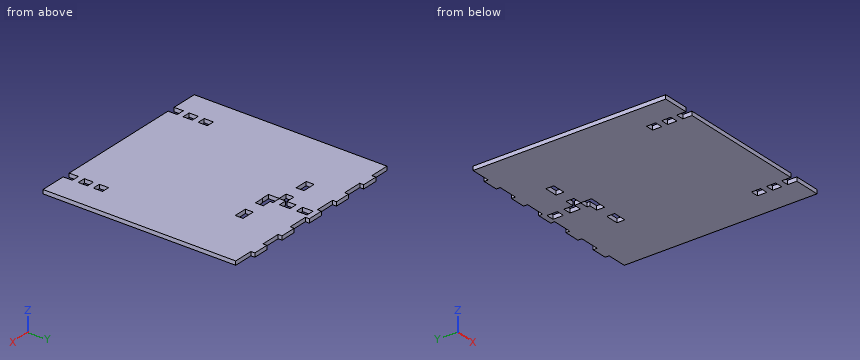
from build123d import *

# Parameters (mm, degrees)
ESQUISSE1_W              = 150
ESQUISSE1_H              = 150
BOSS_EXTRU_1_DEPTH       = 3
ESQUISSE12_W             = 6
ESQUISSE12_H             = 7
ENL_V_MAT_EXTRU_3_DEPTH  = 3
ESQUISSE14_W             = 15
ESQUISSE14_H             = 3
ENL_V_MAT_EXTRU_4_DEPTH  = 3
ESQUISSE15_W             = 10
ESQUISSE15_H             = 6
ESQUISSE15_W_2           = 6
ESQUISSE15_H_2           = 8
ESQUISSE15_W_3           = 7
ENL_V_MAT_EXTRU_9_DEPTH  = 10
ESQUISSE17_W             = 6.4
ESQUISSE17_H             = 8.4
ENL_V_MAT_EXTRU_12_DEPTH = 10


with BuildPart() as part:
    # Esquisse1 → Boss.-Extru.1 (new body)
    with BuildSketch(Plane.XY):
        with Locations((75, -75)):
            Rectangle(ESQUISSE1_W, ESQUISSE1_H)
    extrude(amount=BOSS_EXTRU_1_DEPTH)

    # Esquisse12 → Enlèv. mat.-Extru.3 (cut)
    with BuildSketch(Plane(origin=(0, 0, 0), x_dir=(-1, 0, 0), z_dir=(0, 0, -1))):
        with Locations((-127, -123.5)):
            Rectangle(ESQUISSE12_W, ESQUISSE12_H)
        with Locations((-127, -135)):
            Rectangle(ESQUISSE12_W, ESQUISSE12_H)
        with Locations((-127, -146.5)):
            Rectangle(ESQUISSE12_W, ESQUISSE12_H)
        with Locations((-23, -123.5)):
            Rectangle(ESQUISSE12_W, ESQUISSE12_H)
        with Locations((-23, -135)):
            Rectangle(ESQUISSE12_W, ESQUISSE12_H)
        with Locations((-23, -146.5)):
            Rectangle(ESQUISSE12_W, ESQUISSE12_H)
    extrude(amount=-ENL_V_MAT_EXTRU_3_DEPTH, mode=Mode.SUBTRACT)

    # Esquisse14 → Enlèv. mat.-Extru.4 (cut)
    with BuildSketch(Plane(origin=(0, 0, 0), x_dir=(-1, 0, 0), z_dir=(0, 0, -1))):
        with Locations((-142.5, -1.5)):
            Rectangle(ESQUISSE14_W, ESQUISSE14_H)
        with Locations((-115.5, -1.5)):
            Rectangle(ESQUISSE14_W, ESQUISSE14_H)
        with Locations((-88.5, -1.5)):
            Rectangle(ESQUISSE14_W, ESQUISSE14_H)
        with Locations((-61.5, -1.5)):
            Rectangle(ESQUISSE14_W, ESQUISSE14_H)
        with Locations((-34.5, -1.5)):
            Rectangle(ESQUISSE14_W, ESQUISSE14_H)
        with Locations((-7.5, -1.5)):
            Rectangle(ESQUISSE14_W, ESQUISSE14_H)
    extrude(amount=-ENL_V_MAT_EXTRU_4_DEPTH, mode=Mode.SUBTRACT)

    # Esquisse15 → Enlèv. mat.-Extru.9 (cut)
    with BuildSketch(Plane(origin=(0, 0, 0), x_dir=(-1, 0, 0), z_dir=(0, 0, -1))):
        with Locations((-50, -27)):
            Rectangle(ESQUISSE15_W, ESQUISSE15_H)
        Polygon((-78, -17), (-78, -25), (-72, -25), (-72, -30), (-65, -30), (-65, -24), (-72, -24), (-72, -17), align=None)
        with Locations((-75, -8)):
            Rectangle(ESQUISSE15_W_2, ESQUISSE15_H_2)
        with Locations((-81.5, -35)):
            Rectangle(ESQUISSE15_W_3, ESQUISSE15_H)
        with Locations((-100, -35)):
            Rectangle(ESQUISSE15_W, ESQUISSE15_H)
    extrude(amount=-ENL_V_MAT_EXTRU_9_DEPTH, mode=Mode.SUBTRACT)

    # Esquisse17 → Enlèv. mat.-Extru.12 (cut)
    with BuildSketch(Plane(origin=(0, 0, 0), x_dir=(-1, 0, 0), z_dir=(0, 0, -1))):
        with Locations((-75, -34)):
            Rectangle(ESQUISSE17_W, ESQUISSE17_H)
    extrude(amount=-ENL_V_MAT_EXTRU_12_DEPTH, mode=Mode.SUBTRACT)


solid = part.part
Read the model definition and answer for the solid it produces. Units are mm, in the model's axes. Round coordinates to 2 decimals unless told otherwise and drop trailing zeros. Write each loop counter-clockwise with the first axis right and the second up, starting at its lowest first coordinate (ties: lowest second). Pieces come first, ordered by that corner, then holes.
1. The part is cut by section C-C, the plane x = 138. Determine the outline of the cut face in (y, z).
2. Straight lines are drawn through the part: L1, parallel to X at y = -37, z = 1.2; L2, parallel to X at y = -9.5, z = 2.75; L3, parallel to X at y = -137, z = 1.85. For each, find the intervals that lie inside material, in ascending order.
3. Given pin 1 Ø1.5 at (x, z) = (83, 1) entering from +Y, flat-ended and moving along its own axis, determine where the tip first touches the part or whether it passes through.
4. The part is cut by section A-A, the plane x = 47.5. Determine the outline of the cut face in (y, z).
5. The part is cut by section B-B, the plane z = 2.35. State how many separate pieces and enclosed holes the cut face has, then the cut area to 3 significant figures.
Values:
1. outline: (-150, 0) - (-3, 0) - (-3, 3) - (-150, 3) - close
2. L1: x = 0 to 71.8, 85 to 95, 105 to 150
2. L2: x = 0 to 72, 78 to 150
2. L3: x = 0 to 20, 26 to 124, 130 to 150
3. pin 1: stops at y = -3
4. outline: (-150, 0) - (-30, 0) - (-30, 3) - (-150, 3) - close; (-24, 0) - (0, 0) - (0, 3) - (-24, 3) - close
5. separate pieces: 1
5. enclosed holes: 8
5. area: 21,600 mm2
